```python
from build123d import *

# Parameters (mm, degrees)
SKETCH1_R           = 3.5
BOSS_EXTRUDE1_DEPTH = 3.175


with BuildPart() as part:
    # Sketch1 → Boss-Extrude1 (new body)
    with BuildSketch(Plane(origin=(0, 0, 0), x_dir=(1, 0, 0), z_dir=(0, 1, 0))):
        with BuildLine():
            Line((-152.4, 19.05), (-107.95, 19.05))
            ThreePointArc((-107.95, 19.05), (-76.519103576, 6.030896424), (-63.5, -25.4))
            Line((-63.5, -25.4), (-25.4, -25.4))
            Line((-25.4, -25.4), (-25.4, -28.575))
            Line((-25.4, -28.575), (-63.5, -28.575))
            Line((-63.5, -28.575), (-63.5, -31.75))
            Line((-63.5, -31.75), (63.5, -31.75))
            Line((63.5, -31.75), (63.5, -28.575))
            Line((63.5, -28.575), (25.4, -28.575))
            Line((25.4, -28.575), (25.4, -25.4))
            Line((25.4, -25.4), (63.5, -25.4))
            ThreePointArc((63.5, -25.4), (76.519103576, 6.030896424), (107.95, 19.05))
            Line((107.95, 19.05), (152.4, 19.05))
            Line((152.4, 19.05), (152.4, 25.4))
            Line((152.4, 25.4), (127, 25.4))
            Line((127, 25.4), (127, 28.575))
            Line((127, 28.575), (101.6, 28.575))
            Line((101.6, 28.575), (101.6, 25.4))
            Line((101.6, 25.4), (-101.6, 25.4))
            Line((-101.6, 25.4), (-101.6, 28.575))
            Line((-101.6, 28.575), (-127, 28.575))
            Line((-127, 28.575), (-127, 25.4))
            Line((-127, 25.4), (-152.4, 25.4))
            Line((-152.4, 25.4), (-152.4, 19.05))
        make_face()
        with Locations((-44.45, -12.7)):
            Circle(SKETCH1_R, mode=Mode.SUBTRACT)
        with Locations((12.7, -12.7)):
            Circle(SKETCH1_R, mode=Mode.SUBTRACT)
        with Locations((44.45, -12.7)):
            Circle(SKETCH1_R, mode=Mode.SUBTRACT)
        with Locations((-44.45, 12.7)):
            Circle(SKETCH1_R, mode=Mode.SUBTRACT)
        with Locations((12.7, 12.7)):
            Circle(SKETCH1_R, mode=Mode.SUBTRACT)
        with Locations((44.45, 12.7)):
            Circle(SKETCH1_R, mode=Mode.SUBTRACT)
    extrude(amount=BOSS_EXTRUDE1_DEPTH)


solid = part.part
```
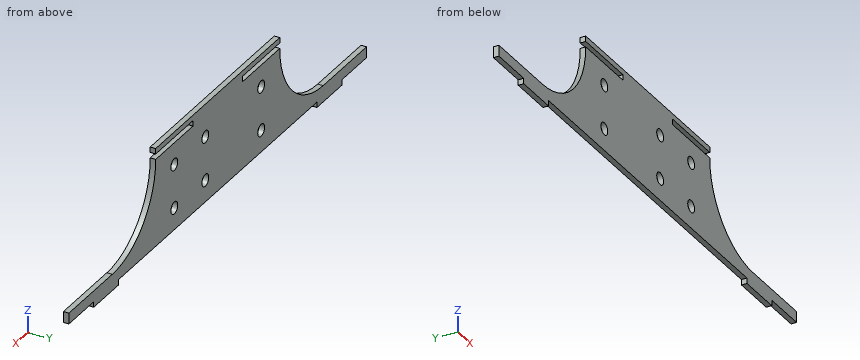
Work out the finished part from the listing and answer in its coordinate system (mm). Coordinates: 2 decimals unless noted, no trailing zeros. Write each loop counter-clockwise with the first axis right and the second up, starting at its lowest first coordinate (ties: lowest second). Pieces come first, ordered by that corner, then holes. Notation, with made-up numbers: (-27.75, 69) - (27.25, 69) arc R21 cw to (27.25, 98) - close; hole circle Ø4 at (6.25, -26.5). An arc over 180 degrees is marked (long way). Answer as a JSON object with one key per item and string values.
Q1. Find section B-B (x = 12.7). Write down the section's boundary in (y, z) (3 decimals), plus the area to 3 significant figures.
Results list:
{"outline": "(0, -25.4) - (3.175, -25.4) - (3.175, -16.2) - (0, -16.2) - close; (0, -9.2) - (3.175, -9.2) - (3.175, 9.2) - (0, 9.2) - close; (0, 16.2) - (3.175, 16.2) - (3.175, 31.75) - (0, 31.75) - close", "area": "137 mm^2"}
Q2. Find section D-D (x = -32.5). Write down the section's boundary in (y, z) (3 decimals).
Results list:
{"outline": "(0, -25.4) - (3.175, -25.4) - (3.175, 25.4) - (0, 25.4) - close; (0, 28.575) - (3.175, 28.575) - (3.175, 31.75) - (0, 31.75) - close"}
Q3. Find section A-A (x = 44.45). Write down the section's boundary in (y, z) (3 decimals).
Results list:
{"outline": "(0, -25.4) - (3.175, -25.4) - (3.175, -16.2) - (0, -16.2) - close; (0, -9.2) - (3.175, -9.2) - (3.175, 9.2) - (0, 9.2) - close; (0, 16.2) - (3.175, 16.2) - (3.175, 25.4) - (0, 25.4) - close; (0, 28.575) - (3.175, 28.575) - (3.175, 31.75) - (0, 31.75) - close"}
Q4. Consider L1, parallel to Z at x = -44.45, y = 2.2 (3 decimals); L2, parallel to Z at x = 12.7, y = 0.6; L3, parallel to X at y = 1.7, z = -12.7. Determine where each line is inside the solid, lowest interval first. Write a range as from..to.
Results list:
{"L1": "z = -25.4..-16.2, -9.2..9.2, 16.2..25.4, 28.575..31.75", "L2": "z = -25.4..-16.2, -9.2..9.2, 16.2..31.75", "L3": "x = -85.05..-47.95, -40.95..9.2, 16.2..40.95, 47.95..85.05"}
Q5. Given pin 1 Ø1 at (y, z) = (0.5, 4.5) entering from -X; pin 2 Ø1.5 at (y, z) = (3, -3) entering from +X, each flat-ended and moving along its own axis, determine where each tip first touches the part or whether it passes through.
Results list:
{"pin 1": "stops at x = -68.99", "pin 2": "stops at x = 74.39"}
Q6. Find section C-C (z = -12.7). Write down the section's boundary in (x, y) (3 decimals), plus the area to 3 significant figures.
Results list:
{"outline": "(-85.055, 0) - (-47.95, 0) - (-47.95, 3.175) - (-85.055, 3.175) - close; (-40.95, 0) - (9.2, 0) - (9.2, 3.175) - (-40.95, 3.175) - close; (16.2, 0) - (40.95, 0) - (40.95, 3.175) - (16.2, 3.175) - close; (47.95, 0) - (85.055, 0) - (85.055, 3.175) - (47.95, 3.175) - close", "area": "473 mm^2"}
